from build123d import *

# Parameters (mm, degrees)
BOSS_EXTRUDE1_DEPTH = 30
CHAMFER1_SIZE       = 12
FILLET1_R           = 2
SKETCH2_W           = 3
SKETCH2_H           = 9.5
CUT_EXTRUDE1_DEPTH  = 30


with BuildPart() as part:
    # Sketch1 → Boss-Extrude1 (new body)
    with BuildSketch(Plane.XY):
        Polygon((6.861356932, 34.926253687), (17.861356932, 34.926253687), (17.861356932, 36.926253687), (-7.138643068, 36.926253687), (-7.138643068, 34.926253687), (3.861356932, 34.926253687), (3.861356932, -5.073746313), (-7.138643068, -5.073746313), (-7.138643068, -7.073746313), (17.861356932, -7.073746313), (17.861356932, -5.073746313), (6.861356932, -5.073746313), align=None)
    extrude(amount=BOSS_EXTRUDE1_DEPTH)

    # Chamfer1
    chamfer1_edges = [part.edges().sort_by_distance(p)[0] for p in [
        (-7.138643068, 35.926253687, 30),
        (17.861356932, 35.926253687, 30),
    ]]
    chamfer(chamfer1_edges, length=CHAMFER1_SIZE)

    # Fillet1
    fillet1_edges = [part.edges().sort_by_distance(p)[0] for p in [
        (3.861356932, -5.073746313, 14.5),
        (3.861356932, 34.926253687, 14.5),
        (6.861356932, 34.926253687, 14.5),
        (6.861356932, -5.073746313, 14.5),
    ]]
    fillet(fillet1_edges, radius=FILLET1_R)

    # Sketch2 → Cut-Extrude1 (cut)
    with BuildSketch(Plane(origin=(0, 36.926253687, 0), x_dir=(1, 0, 0), z_dir=(0, 1, 0))):
        with Locations((-2.045453442, -8.544505852)):
            Rectangle(SKETCH2_W, SKETCH2_H)
    extrude(amount=-CUT_EXTRUDE1_DEPTH, mode=Mode.SUBTRACT)


solid = part.part
Here's how the part is built. I have some questions about the finished solid (model axes, mm). A direction names the side the tool comes from. Round coordinates to 2 decimals unless told otherwise and drop trailing zeros. Loops run counter-clockwise (first coordinate to the right, second up) from the corner with the lowest first, then second, coordinate; pieces in that order, holes last. Notation, with made-up numbers: (-14, 17.5) -> (29, 17.5) arc R16 cw to (29, 34.5) -> close; hole circle Ø10 at (7.5, 20.25). An arc over 180 degrees is marked (long way). Write each question's results on one line, items separated by ' | '.
(1) If I drill on L1, parallel to Y at x = -5.5, z = 16; L2, parallel to X at y = 17, z = 24; L3, parallel to Y at x = 2.75, z = 13, over which ranges is the centre line in solid material (lowest first)?
Worked answers:
L1: -7.07 to -5.07, 34.93 to 36.93 | L2: 3.86 to 6.86 | L3: -7.07 to -4.87, 34.72 to 36.93
(2) If we section it at A-A, the plane z = 8.5: List the corners of the cut face in (x, y) for me.
Worked answers:
outline: (-7.14, -7.07) -> (17.86, -7.07) -> (17.86, -5.07) -> (8.86, -5.07) arc R2 cw to (6.86, -3.07) -> (6.86, 32.93) arc R2 cw to (8.86, 34.93) -> (17.86, 34.93) -> (17.86, 36.93) -> (-0.55, 36.93) -> (-0.55, 34.93) -> (1.86, 34.93) arc R2 cw to (3.86, 32.93) -> (3.86, -3.07) arc R2 cw to (1.86, -5.07) -> (-7.14, -5.07) -> close; (-7.14, 34.93) -> (-3.55, 34.93) -> (-3.55, 36.93) -> (-7.14, 36.93) -> close
(3) If we section it at C-C, the plane y = 1: List the corners of the cut face in (x, z) for me, then the cut area to 3 significant figures.
Worked answers:
outline: (3.86, 0) -> (6.86, 0) -> (6.86, 29) -> (5.86, 30) -> (4.86, 30) -> (3.86, 29) -> close | area: 89.0 mm2
(4) We'd pull the mould along X, two halves only. Please class faces 1 (the face through (6, 36.926, 11)), 2 (the face through (-2, 36, 3.795)), 3 (the face through (3.26, 34.356, 14.703)): released by +X, released by -X, zero draft, split by the parting line, or undercut.
Worked answers:
face 1: zero draft | face 2: undercut | face 3: released by -X
(5) For faces 4 (the face through (4.22, 16.66, 29.36)), 5 (the face through (3.861, 15, 14)), 6 (the face through (5, 15, 0)), 7 (the face through (7.43, -4.47, 14.7)), 8 (the face through (-3.545, 36, 9)), which set-ups out of +Z, -Z, +X, -X, +Y, -Y let a thin tool reach every point of the face, with its end or its side?
Worked answers:
face 4: +Z, -X, +Y, -Y | face 5: +Z, -Z, -X | face 6: -Z, +X, -X, +Y, -Y | face 7: +Z, -Z, +X | face 8: +Y
(6) For P1, Ø1.6, axis at x = -2.5, y = 35.5, coming from the +Z side; P2, Ø6, axis at y = 14.5, z = 9, coming from the -X side; P3, Ø1, axis at y = 3, z = 9.5, coming from the +X side, each with a flat end and sliding along its axis, tell me the tip position at first contact or that it passes through.
Worked answers:
P1: z = 23.44 | P2: x = 3.86 | P3: x = 6.86
(7) If we section it at D-D, the plane z = 2: List the corners of the cut face in (x, y) for me.
Worked answers:
outline: (-7.14, -7.07) -> (17.86, -7.07) -> (17.86, -5.07) -> (8.86, -5.07) arc R2 cw to (6.86, -3.07) -> (6.86, 32.93) arc R2 cw to (8.86, 34.93) -> (17.86, 34.93) -> (17.86, 36.93) -> (-7.14, 36.93) -> (-7.14, 34.93) -> (1.86, 34.93) arc R2 cw to (3.86, 32.93) -> (3.86, -3.07) arc R2 cw to (1.86, -5.07) -> (-7.14, -5.07) -> close
(8) If we section it at B-B, the plane x = 1: List the corners of the cut face in (y, z) for me.
Worked answers:
outline: (-7.07, 0) -> (-5.07, 0) -> (-5.07, 26.14) -> (-7.07, 26.14) -> close; (34.93, 0) -> (36.93, 0) -> (36.93, 26.14) -> (34.93, 26.14) -> close
